Can you work these out from the model? Positions are in its coordinate system, mm. A direction names the side the tool comes from. Round coordinates to 2 decimals unless told otherwise and drop trailing zeros. Write each loop counter-clockwise with the first axis right and the second up, starting at its lowest first coordinate (ties: lowest second). Pieces come first, ordered by that corner, then holes. Notation, with made-up numbers: M -9,60.25 L 26,60.25 A33 ccw 26,99.25 Z; hole C 88,84 d3. An arc over 180 degrees is marked long. Use one line per item in the form item = value. Start each with the question number.
```python
from build123d import *

# Parameters (mm, degrees)
F0_W     = 15
F0_H     = 15.8
F0_R     = 3
F0_R_2   = 1.6
F1_DEPTH = 11
F2_DEPTH = 5
F3_R     = 2
F4_W     = 0.5
F4_H     = 6
F5_DEPTH = 1


with BuildPart() as f1:
    # F0 (on Top) → F1 (new body)
    with BuildSketch(Plane.XY):
        Rectangle(F0_W, F0_H)
        Circle(F0_R, mode=Mode.SUBTRACT)
        Circle(F0_R)
        Circle(F0_R_2, mode=Mode.SUBTRACT)
    extrude(amount=F1_DEPTH)

    # F0 (on Top) → F2 (cut)
    with BuildSketch(Plane.XY):
        Circle(F0_R)
        Circle(F0_R_2, mode=Mode.SUBTRACT)
    extrude(amount=F2_DEPTH, mode=Mode.SUBTRACT)

    # F3
    f3_edges = [f1.edges().sort_by_distance(p)[0] for p in [
        (-7.5, 7.9, 5.5),
        (-7.5, -7.9, 5.5),
        (7.5, -7.9, 5.5),
        (7.5, 7.9, 5.5),
    ]]
    fillet(f3_edges, radius=F3_R)

    # F4 (on face) → F5 (cut)
    with BuildSketch(Plane.XY.offset(11)):
        with Locations((-0.25, 4.9)):
            Rectangle(F4_W, F4_H)
        with Locations((0.25, 4.9)):
            Rectangle(F4_W, F4_H)
        Polygon((2, 7.9), (1.5, 7.9), (1.5, 1.9), (2, 1.9), (2.5, 1.9), (2.5, 7.9), align=None)
        Polygon((4, 7.9), (3.5, 7.9), (3.5, 1.9), (4, 1.9), (4.5, 1.9), (4.5, 7.9), align=None)
        with BuildLine():
            ThreePointArc((6.5, 7.632051), (6.017638, 7.831852), (5.5, 7.9))
            Line((5.5, 7.9), (5.5, 1.9))
            Line((5.5, 1.9), (6, 1.9))
            Line((6, 1.9), (6.5, 1.9))
            Line((6.5, 1.9), (6.5, 7.632051))
        make_face()
        Polygon((-1.5, 1.9), (-1.5, 7.9), (-2, 7.9), (-2.5, 7.9), (-2.5, 1.9), (-2, 1.9), align=None)
        Polygon((-3.5, 1.9), (-3.5, 7.9), (-4, 7.9), (-4.5, 7.9), (-4.5, 1.9), (-4, 1.9), align=None)
        with BuildLine():
            Line((-5.5, 1.9), (-5.5, 7.9))
            ThreePointArc((-5.5, 7.9), (-6.017638, 7.831852), (-6.5, 7.632051))
            Line((-6.5, 7.632051), (-6.5, 1.9))
            Line((-6.5, 1.9), (-6, 1.9))
            Line((-6, 1.9), (-5.5, 1.9))
        make_face()
        with BuildLine():
            Line((-6.5, -1.9), (-6.5, -7.632051))
            ThreePointArc((-6.5, -7.632051), (-6.017638, -7.831852), (-5.5, -7.9))
            Line((-5.5, -7.9), (-5.5, -1.9))
            Line((-5.5, -1.9), (-6, -1.9))
            Line((-6, -1.9), (-6.5, -1.9))
        make_face()
        Polygon((-4.5, -1.9), (-4.5, -7.9), (-4, -7.9), (-3.5, -7.9), (-3.5, -1.9), (-4, -1.9), align=None)
        Polygon((-2.5, -1.9), (-2.5, -7.9), (-2, -7.9), (-1.5, -7.9), (-1.5, -1.9), (-2, -1.9), align=None)
        Polygon((0, -7.9), (0.5, -7.9), (0.5, -1.9), (0, -1.9), (-0.5, -1.9), (-0.5, -7.9), align=None)
        Polygon((2, -7.9), (2.5, -7.9), (2.5, -1.9), (2, -1.9), (1.5, -1.9), (1.5, -7.9), align=None)
        Polygon((4, -7.9), (4.5, -7.9), (4.5, -1.9), (4, -1.9), (3.5, -1.9), (3.5, -7.9), align=None)
        with BuildLine():
            ThreePointArc((5.5, -7.9), (6.017638, -7.831852), (6.5, -7.632051))
            Line((6.5, -7.632051), (6.5, -1.9))
            Line((6.5, -1.9), (6, -1.9))
            Line((6, -1.9), (5.5, -1.9))
            Line((5.5, -1.9), (5.5, -7.9))
        make_face()
    extrude(amount=-F5_DEPTH, mode=Mode.SUBTRACT)


solid = f1.part
```
1. If we section it at B-B (x = 0): List the corners of the cut face in (y, z) for me.
2. Please list where these lines run through material, in increasing order: line 1 along Y through (x, z) = (0, 1.1); line 2 along Y through (x, z) = (0, 7.25); line 3 along Z through (x, y) = (6, -4).
3. Will these pins go through, and if not, where does the flat tip stop? pin 1 (0.5 mm diameter, centred on x = 4, z = 10.5, fed in from -Y); pin 2 (0.5 mm diameter, centred on x = 0, y = -4.5, fed in from +Z); pin 3 (0.5 mm diameter, centred on y = 6.5, z = 10.5, fed in from +X).
4. If we section it at A-A (y = 0): List the corners of the cut face in (x, z) for me.
5. Which directions (+Z, -Z, +X, -X, +Y, -Y) give clear straight access to the entire face, cutting with the end or side of a thin tool? Please do faces 1 (the face through (5.5, 4.9, 10.5)), 2 (the face through (1.3, -1.3, 5)), 3 (the face through (1.5, -4.9, 10.5)).
6. If we section it at C-C (z = 3.5): List the corners of the cut face in (x, y) for me, and give its area (3 significant figures).
7. If we section it at D-D (x = -4.25): List the corners of the cut face in (y, z) for me.
Model answer:
q1.outline = M -7.9,0 L -3,0 L -3,5 L -1.6,5 L -1.6,11 L -1.9,11 L -1.9,10 L -7.9,10 Z; M 1.6,5 L 3,5 L 3,0 L 7.9,0 L 7.9,10 L 1.9,10 L 1.9,11 L 1.6,11 Z
q2.line_1 = -7.9 to -3, 3 to 7.9
q2.line_2 = -7.9 to -1.6, 1.6 to 7.9
q2.line_3 = 0 to 10
q3.pin_1 = -1.9
q3.pin_2 = 10
q3.pin_3 = 7.47
q4.outline = M -7.5,0 L -3,0 L -3,5 L -1.6,5 L -1.6,11 L -7.5,11 Z; M 1.6,5 L 3,5 L 3,0 L 7.5,0 L 7.5,11 L 1.6,11 Z
q5.face_1 = +Z, +Y
q5.face_2 = -Z
q5.face_3 = +Z, -Y
q6.outline = M -7.5,-5.9 A2 ccw -5.5,-7.9 L 5.5,-7.9 A2 ccw 7.5,-5.9 L 7.5,5.9 A2 ccw 5.5,7.9 L -5.5,7.9 A2 ccw -7.5,5.9 Z; hole C 0,0 d6
q6.area = 205 mm2
q7.outline = M -7.9,0 L 7.9,0 L 7.9,10 L 1.9,10 L 1.9,11 L -1.9,11 L -1.9,10 L -7.9,10 Z
